For this review, take the finished solid that the model builds, in its own axes (mm). A direction names the side the tool comes from. Round coordinates to 2 decimals unless told otherwise and drop trailing zeros. Write each loop counter-clockwise with the first axis right and the second up, starting at its lowest first coordinate (ties: lowest second). Pieces come first, ordered by that corner, then holes. Notation, with made-up numbers: (43, 61.5) -> (98, 61.5) arc R11 cw to (98, 80.5) -> close; hole circle Ø3 at (42, 6). An arc over 180 degrees is marked (long way). Answer in a Markdown table with one row per item.
from build123d import *

# Parameters (mm, degrees)
SKETCH187_W     = 50
SKETCH187_H     = 50
PAD032_DEPTH    = 20
POCKET156_DEPTH = 20.001
POCKET157_DEPTH = 50.001
POCKET158_DEPTH = 50.001
SKETCH191_R     = 1.55
POCKET159_DEPTH = 5


with BuildPart() as part:
    # Sketch187 → Pad032 (new body)
    with BuildSketch(Plane.XY):
        Rectangle(SKETCH187_W, SKETCH187_H)
    extrude(amount=PAD032_DEPTH)

    # Sketch188 (on Face6 of Pad032) → Pocket156 (cut, through all)
    with BuildSketch(Plane.XY.offset(20)):
        with BuildLine():
            Line((-18, 15), (-17, 15))
            ThreePointArc((-17, 15), (-15.585786, 15.585786), (-15, 17))
            Line((-15, 17), (-15, 18))
            ThreePointArc((-13, 20), (-14.414214, 19.414214), (-15, 18))
            Line((-13, 20), (13, 20))
            ThreePointArc((15, 18), (14.414214, 19.414214), (13, 20))
            Line((15, 18), (15, 17))
            ThreePointArc((15, 17), (15.585786, 15.585786), (17, 15))
            Line((17, 15), (18, 15))
            ThreePointArc((20, 13), (19.414214, 14.414214), (18, 15))
            Line((20, 13), (20, -13))
            ThreePointArc((18, -15), (19.414214, -14.414214), (20, -13))
            Line((18, -15), (17, -15))
            ThreePointArc((17, -15), (15.585786, -15.585786), (15, -17))
            Line((15, -17), (15, -18))
            ThreePointArc((13, -20), (14.414214, -19.414214), (15, -18))
            Line((13, -20), (-13, -20))
            ThreePointArc((-15, -18), (-14.414214, -19.414214), (-13, -20))
            Line((-15, -18), (-15, -17))
            ThreePointArc((-15, -17), (-15.585786, -15.585786), (-17, -15))
            Line((-17, -15), (-18, -15))
            ThreePointArc((-20, -13), (-19.414214, -14.414214), (-18, -15))
            Line((-20, -13), (-20, 13))
            ThreePointArc((-18, 15), (-19.414214, 14.414214), (-20, 13))
        make_face()
    extrude(amount=-POCKET156_DEPTH, mode=Mode.SUBTRACT)

    # Sketch189 (on Face3 of Pocket156) → Pocket157 (cut, through all)
    with BuildSketch(Plane.YZ.offset(25)):
        with BuildLine():
            Line((-15, 10), (15, 10))
            ThreePointArc((20, 5), (18.535534, 8.535534), (15, 10))
            Line((20, 5), (20, 0))
            Line((20, 0), (-20, 0))
            Line((-20, 0), (-20, 5))
            ThreePointArc((-15, 10), (-18.535534, 8.535534), (-20, 5))
        make_face()
    extrude(amount=-POCKET157_DEPTH, mode=Mode.SUBTRACT)

    # Sketch190 (on Face6 of Pocket156) → Pocket158 (cut, through all)
    with BuildSketch(Plane.XZ.offset(25)):
        with BuildLine():
            Line((-15, 10), (15, 10))
            ThreePointArc((20, 5), (18.535534, 8.535534), (15, 10))
            Line((20, 5), (20, 0))
            Line((20, 0), (-20, 0))
            Line((-20, 0), (-20, 5))
            ThreePointArc((-15, 10), (-18.535534, 8.535534), (-20, 5))
        make_face()
    extrude(amount=-POCKET158_DEPTH, mode=Mode.SUBTRACT)

    # Sketch191 → Pocket159 (cut)
    with BuildSketch(Plane.XY.offset(20)):
        with Locations((-20, 20)):
            Circle(SKETCH191_R)
        with Locations((20, 20)):
            Circle(SKETCH191_R)
        with Locations((20, -20)):
            Circle(SKETCH191_R)
        with Locations((-20, -20)):
            Circle(SKETCH191_R)
    extrude(amount=-POCKET159_DEPTH, mode=Mode.SUBTRACT)


with BuildPart() as part_1:
    # Body033 placement: moved
    add(part.part.moved(Location((85, 85, 0))))


solid = part_1.part
1) Consider section A-A on y = 95. State the section outline as (x, z) points, then the cut area to 3 significant figures.
Solved:
| item | result |
|---|---|
| outline | (60, 10) -> (65, 10) -> (65, 20) -> (60, 20) -> close; (105, 10) -> (110, 10) -> (110, 20) -> (105, 20) -> close |
| area | 100 mm² |
2) Mouldability with a two-part tool opening along X and no side actions: class faces 1 (the flat face through (107, 85, 20)), 2 (the cylindrical face through (66.478, 65.466, 17.535)), 3 (the cylindrical face through (69.4, 100.57, 15.05)) as pulls with the +X half, pulls with the -X half, needs draft (parallel to the pull), parting line crosses it, or undercut.
Solved:
| item | result |
|---|---|
| face 1 | needs draft |
| face 2 | undercut |
| face 3 | undercut |
3) Clearance check with flat-ended pins moving along their axes: pin 1 Ø1.5 at (x, y) = (65, 65) entering from +Z; pin 2 Ø7.5 at (x, y) = (65, 90) entering from -Z. State where each tip first meets the part, or that it passes through.
Solved:
| item | result |
|---|---|
| pin 1 | z = 15 |
| pin 2 | z = 10 |
4) Consider section C-C on z = 17. State how many separate pieces and enclosed holes the cut face has, then the cut area to 3 significant figures.
Solved:
| item | result |
|---|---|
| separate pieces | 1 |
| enclosed holes | 5 |
| area | 973 mm² |
5) Consider section B-B on z = 12. State the section outline as (x, y) points.
Solved:
| item | result |
|---|---|
| outline | (60, 60) -> (110, 60) -> (110, 110) -> (60, 110) -> close; hole (65, 72) arc R2 ccw to (67, 70) -> (68, 70) arc R2 cw to (70, 68) -> (70, 67) arc R2 ccw to (72, 65) -> (98, 65) arc R2 ccw to (100, 67) -> (100, 68) arc R2 cw to (102, 70) -> (103, 70) arc R2 ccw to (105, 72) -> (105, 98) arc R2 ccw to (103, 100) -> (102, 100) arc R2 cw to (100, 102) -> (100, 103) arc R2 ccw to (98, 105) -> (72, 105) arc R2 ccw to (70, 103) -> (70, 102) arc R2 cw to (68, 100) -> (67, 100) arc R2 ccw to (65, 98) -> close |
6) For faces 4 (the flat face through (63, 65, 2)), 5 (the flat face through (85, 105, 15)), 6 (the cylindrical face through (66.432, 104.406, 17.535)), 7 (the flat face through (65, 107, 2)), list the 3-axis set-ups (+Z, -Z, +X, -X, +Y, -Y) from which the entire face can be reached by the end or side of a thin tool; tool diameter is ignored.
Solved:
| item | result |
|---|---|
| face 4 | -Z, +X, -X |
| face 5 | +Z, -Z |
| face 6 | +Z |
| face 7 | -Z, +Y, -Y |
7) For line 1 (Y direction, x = 81.5, z = 14.75); line 2 (Z direction, x = 73, y = 106); line 3 (X direction, y = 99.5, z = 17.5), list the stretches that pass through material, from the lowest coordinate up. Write a range as [from, to].
Solved:
| item | result |
|---|---|
| line 1 | [60, 65], [105, 110] |
| line 2 | [10, 20] |
| line 3 | [60, 65.68], [104.32, 110] |
